The listing builds one solid part. Answer for the finished solid, in the listing's coordinates (mm). Coordinates: 2 decimals unless noted, no trailing zeros. Write each loop counter-clockwise with the first axis right and the second up, starting at its lowest first coordinate (ties: lowest second). Pieces come first, ordered by that corner, then holes. Notation, with made-up numbers: M 33.25,12.25 L 72.25,12.25 A31 cw 72.25,45.25 Z; hole C 20.25,77.25 d2. An arc over 180 degrees is marked long. Answer as CSV lines item,"result".
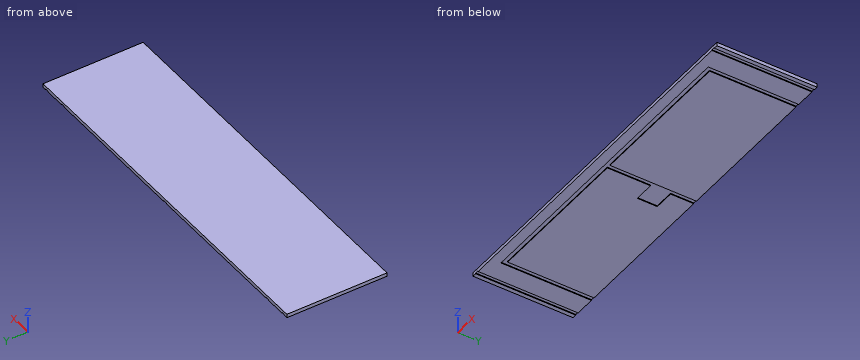
```python
from build123d import *

# Parameters (mm, degrees)
F1_W     = 20
F1_H     = 500
F1_W_2   = 18
F1_W_3   = 752
F1_H_2   = 431.6755512357
F2_DEPTH = 18
F3_DEPTH = 4


with BuildPart() as f2:
    # F1 (on Top) → F2 (new body)
    with BuildSketch(Plane.XY):
        with Locations((10, 250)):
            Rectangle(F1_W, F1_H)
        with Locations((29, 250)):
            Rectangle(F1_W_2, F1_H)
        Polygon((38, 500), (38, 0), (1802, 0), (1802, 500), (1702, 500), (1702, 68.3244487643), (1702, 48.3244487643), (138, 48.3244487643), (138, 68.3244487643), (138, 500), align=None)
        with Locations((1811, 250)):
            Rectangle(F1_W_2, F1_H)
        Polygon((158, 500), (138, 500), (138, 68.3244487643), (138, 48.3244487643), (1702, 48.3244487643), (1702, 68.3244487643), (1702, 500), (1682, 500), (1682, 68.3244487643), (930, 68.3244487643), (930, 500), (910, 500), (910, 384.1622243822), (810, 384.1622243822), (810, 284.1622243822), (910, 284.1622243822), (910, 68.3244487643), (158, 68.3244487643), align=None)
        with Locations((1830, 250)):
            Rectangle(F1_W, F1_H)
        Polygon((910, 500), (158, 500), (158, 68.3244487643), (910, 68.3244487643), (910, 284.1622243822), (810, 284.1622243822), (810, 384.1622243822), (910, 384.1622243822), align=None)
        with Locations((1306, 284.1622243822)):
            Rectangle(F1_W_3, F1_H_2)
    extrude(amount=F2_DEPTH)

    # F1 (on Top) → F3 (cut)
    with BuildSketch(Plane.XY):
        Polygon((158, 500), (138, 500), (138, 68.3244487643), (138, 48.3244487643), (1702, 48.3244487643), (1702, 68.3244487643), (1702, 500), (1682, 500), (1682, 68.3244487643), (930, 68.3244487643), (930, 500), (910, 500), (910, 384.1622243822), (810, 384.1622243822), (810, 284.1622243822), (910, 284.1622243822), (910, 68.3244487643), (158, 68.3244487643), align=None)
        with Locations((29, 250)):
            Rectangle(F1_W_2, F1_H)
        with Locations((1811, 250)):
            Rectangle(F1_W_2, F1_H)
    extrude(amount=F3_DEPTH, mode=Mode.SUBTRACT)


solid = f2.part
```
Q1. Find section A-A (y = 356.5). Give the vertices of the cut face in (x, z), and give its area (3 significant figures).
Output:
outline,"M 0,0 L 20,0 L 20,4 L 38,4 L 38,0 L 138,0 L 138,4 L 158,4 L 158,0 L 810,0 L 810,4 L 930,4 L 930,0 L 1682,0 L 1682,4 L 1702,4 L 1702,0 L 1802,0 L 1802,4 L 1820,4 L 1820,0 L 1840,0 L 1840,18 L 0,18 Z"
area,"32,300 mm2"
Q2. A flat-ended cylindrical pin translates along its axis: pin 1 Ø14.5 at (x, y) = (1810, 161) entering from -Z. Find the tip coordinate at first contact, or state that the pin passes through.
Output:
pin 1,"z = 4"
Q3. Straight lines are drawn through the part: line 1 (X direction, y = 151.5, z = 3); line 2 (Y direction, x = 907.5, z = 1); line 3 (Y direction, x = 534, z = 2.75). For each, find the intervals that lie inside material, in ascending order.
Output:
line 1,"0 to 20, 38 to 138, 158 to 910, 930 to 1682, 1702 to 1802, 1820 to 1840"
line 2,"0 to 48.32, 68.32 to 284.16, 384.16 to 500"
line 3,"0 to 48.32, 68.32 to 500"
